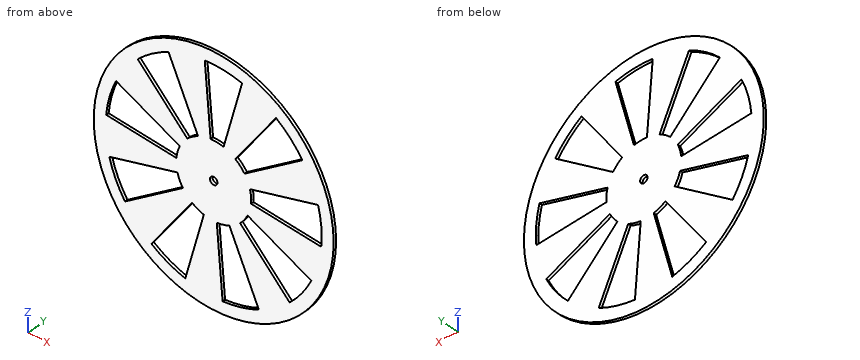
```python
from build123d import *

# Parameters (mm, degrees)
F0_R     = 50.8
F0_R_2   = 1.5875
F1_DEPTH = 1.1938


with BuildPart() as f1:
    # F0 (on Front) → F1 (new body)
    with BuildSketch(Plane.XZ):
        Circle(F0_R)
        with BuildLine():
            ThreePointArc((44.21609, 11.629953), (45.342464, 5.863394), (45.72, 0))
            ThreePointArc((45.72, 0), (45.671777, -2.09932), (45.527211, -4.194212))
            ThreePointArc((45.527211, -4.194212), (44.107234, -12.03621), (41.34708, -19.512494))
            ThreePointArc((41.34708, -19.512494), (37.330616, -26.3959), (32.17988, -32.47728))
            ThreePointArc((32.17988, -32.47728), (26.051375, -37.571855), (19.131311, -41.524828))
            ThreePointArc((19.131311, -41.524828), (11.629953, -44.21609), (3.775225, -45.563868))
            ThreePointArc((3.775225, -45.563868), (-4.194212, -45.527211), (-12.03621, -44.107234))
            ThreePointArc((-12.03621, -44.107234), (-19.512494, -41.34708), (-26.3959, -37.330616))
            ThreePointArc((-26.3959, -37.330616), (-32.47728, -32.17988), (-37.571855, -26.051375))
            ThreePointArc((-37.571855, -26.051375), (-41.524828, -19.131311), (-44.21609, -11.629953))
            ThreePointArc((-44.21609, -11.629953), (-45.563868, -3.775225), (-45.527211, 4.194212))
            ThreePointArc((-45.527211, 4.194212), (-44.107234, 12.03621), (-41.34708, 19.512494))
            ThreePointArc((-41.34708, 19.512494), (-37.330616, 26.3959), (-32.17988, 32.47728))
            ThreePointArc((-32.17988, 32.47728), (-26.051375, 37.571855), (-19.131311, 41.524828))
            ThreePointArc((-19.131311, 41.524828), (-11.629953, 44.21609), (-3.775225, 45.563868))
            ThreePointArc((-3.775225, 45.563868), (4.194212, 45.527211), (12.03621, 44.107234))
            ThreePointArc((12.03621, 44.107234), (19.512494, 41.34708), (26.3959, 37.330616))
            ThreePointArc((26.3959, 37.330616), (32.47728, 32.17988), (37.571855, 26.051375))
            ThreePointArc((37.571855, 26.051375), (41.524828, 19.131311), (44.21609, 11.629953))
        make_face(mode=Mode.SUBTRACT)
        with BuildLine():
            Line((-15.80806, 1.456324), (-45.527211, 4.194212))
            ThreePointArc((-45.527211, 4.194212), (-45.563868, -3.775225), (-44.21609, -11.629953))
            Line((-44.21609, -11.629953), (-15.352809, -4.038178))
            ThreePointArc((-15.352809, -4.038178), (-15.820788, -1.310842), (-15.80806, 1.456324))
        make_face()
        with BuildLine():
            Line((-11.173569, 11.276833), (-32.17988, 32.47728))
            ThreePointArc((-32.17988, 32.47728), (-37.330616, 26.3959), (-41.34708, 19.512494))
            Line((-41.34708, 19.512494), (-14.356625, 6.775171))
            ThreePointArc((-14.356625, 6.775171), (-12.962019, 9.165243), (-11.173569, 11.276833))
        make_face()
        with BuildLine():
            Line((-1.310842, 15.820788), (-3.775225, 45.563868))
            ThreePointArc((-3.775225, 45.563868), (-11.629953, 44.21609), (-19.131311, 41.524828))
            Line((-19.131311, 41.524828), (-6.642816, 14.418343))
            ThreePointArc((-6.642816, 14.418343), (-4.038178, 15.352809), (-1.310842, 15.820788))
        make_face()
        with BuildLine():
            Line((9.165243, 12.962019), (26.3959, 37.330616))
            ThreePointArc((26.3959, 37.330616), (19.512494, 41.34708), (12.03621, 44.107234))
            Line((12.03621, 44.107234), (4.17924, 15.315012))
            ThreePointArc((4.17924, 15.315012), (6.775171, 14.356625), (9.165243, 12.962019))
        make_face()
        with BuildLine():
            Line((15.352809, 4.038178), (44.21609, 11.629953))
            ThreePointArc((44.21609, 11.629953), (41.524828, 19.131311), (37.571855, 26.051375))
            Line((37.571855, 26.051375), (13.045783, 9.045616))
            ThreePointArc((13.045783, 9.045616), (14.418343, 6.642816), (15.352809, 4.038178))
        make_face()
        with BuildLine():
            ThreePointArc((41.34708, -19.512494), (44.107234, -12.03621), (45.527211, -4.194212))
            Line((45.527211, -4.194212), (15.80806, -1.456324))
            ThreePointArc((15.80806, -1.456324), (15.315012, -4.17924), (14.356625, -6.775171))
            Line((14.356625, -6.775171), (41.34708, -19.512494))
        make_face()
        with BuildLine():
            ThreePointArc((19.131311, -41.524828), (26.051375, -37.571855), (32.17988, -32.47728))
            Line((32.17988, -32.47728), (11.173569, -11.276833))
            ThreePointArc((11.173569, -11.276833), (9.045616, -13.045783), (6.642816, -14.418343))
            Line((6.642816, -14.418343), (19.131311, -41.524828))
        make_face()
        with BuildLine():
            ThreePointArc((-12.03621, -44.107234), (-4.194212, -45.527211), (3.775225, -45.563868))
            Line((3.775225, -45.563868), (1.310842, -15.820788))
            ThreePointArc((1.310842, -15.820788), (-1.456324, -15.80806), (-4.17924, -15.315012))
            Line((-4.17924, -15.315012), (-12.03621, -44.107234))
        make_face()
        with BuildLine():
            ThreePointArc((-37.571855, -26.051375), (-32.47728, -32.17988), (-26.3959, -37.330616))
            Line((-26.3959, -37.330616), (-9.165243, -12.962019))
            ThreePointArc((-9.165243, -12.962019), (-11.276833, -11.173569), (-13.045783, -9.045616))
            Line((-13.045783, -9.045616), (-37.571855, -26.051375))
        make_face()
        with BuildLine():
            ThreePointArc((15.875, 0), (15.743911, 2.035901), (15.352809, 4.038178))
            ThreePointArc((15.352809, 4.038178), (14.418343, 6.642816), (13.045783, 9.045616))
            ThreePointArc((13.045783, 9.045616), (11.276833, 11.173569), (9.165243, 12.962019))
            ThreePointArc((9.165243, 12.962019), (6.775171, 14.356625), (4.17924, 15.315012))
            ThreePointArc((4.17924, 15.315012), (1.456324, 15.80806), (-1.310842, 15.820788))
            ThreePointArc((-1.310842, 15.820788), (-4.038178, 15.352809), (-6.642816, 14.418343))
            ThreePointArc((-6.642816, 14.418343), (-9.045616, 13.045783), (-11.173569, 11.276833))
            ThreePointArc((-11.173569, 11.276833), (-12.962019, 9.165243), (-14.356625, 6.775171))
            ThreePointArc((-14.356625, 6.775171), (-15.315012, 4.17924), (-15.80806, 1.456324))
            ThreePointArc((-15.80806, 1.456324), (-15.820788, -1.310842), (-15.352809, -4.038178))
            ThreePointArc((-15.352809, -4.038178), (-14.418343, -6.642816), (-13.045783, -9.045616))
            ThreePointArc((-13.045783, -9.045616), (-11.276833, -11.173569), (-9.165243, -12.962019))
            ThreePointArc((-9.165243, -12.962019), (-6.775171, -14.356625), (-4.17924, -15.315012))
            ThreePointArc((-4.17924, -15.315012), (-1.456324, -15.80806), (1.310842, -15.820788))
            ThreePointArc((1.310842, -15.820788), (4.038178, -15.352809), (6.642816, -14.418343))
            ThreePointArc((6.642816, -14.418343), (9.045616, -13.045783), (11.173569, -11.276833))
            ThreePointArc((11.173569, -11.276833), (12.962019, -9.165243), (14.356625, -6.775171))
            ThreePointArc((14.356625, -6.775171), (15.315012, -4.17924), (15.80806, -1.456324))
            ThreePointArc((15.80806, -1.456324), (15.858256, -0.728931), (15.875, 0))
        make_face()
        Circle(F0_R_2, mode=Mode.SUBTRACT)
    extrude(amount=F1_DEPTH)


solid = f1.part
```
Part model, mm, in its own coordinate system. Round coordinates to 2 decimals unless told otherwise and drop trailing zeros. Order: outer loops, then holes, each group sorted by start corner. A loop starts at its lowest first (then second) coordinate and runs counter-clockwise, first axis right, second up. Notation, with made-up numbers: M 12,28 L 23,28 A8 ccw 23,41 Z; hole C -14,8 d8. An arc over 180 degrees is marked long. Answer in a Markdown table with one row per item. Add a question column.
Q1. Cut at D-D on z = 29.5. Give the cut face in (x, y).
Q2. Cut at B-B on z = -28. Give the cut face in (x, y).
Q3. Cut at C-C on y = -0.7. Give the number of separate pieces and of enclosed holes in the cut face, and give its area (3 significant figures).
Q4. Cut at A-A on x = 0. Give the cut face in (y, z) (1 decimal).
Q5. Wall check: L1, parallel to Z at x = 0, y = -0.3 (1 decimal); L2, parallel to X at y = -0.05, z = 12; L3, parallel to Z at x = -36, y = -1.1. Give the ranges that are in metal, low to high. Write a range as from..to.
Established:
| question | item | result |
|---|---|---|
| 1 | outline | M -41.36,-1.19 L -29.23,-1.19 L -29.23,0 L -41.36,0 Z; M -13.59,-1.19 L -2.44,-1.19 L -2.44,0 L -13.59,0 Z; M 8.05,-1.19 L 20.86,-1.19 L 20.86,0 L 8.05,0 Z; M 34.93,-1.19 L 41.36,-1.19 L 41.36,0 L 34.93,0 Z |
| 2 | outline | M -42.39,-1.19 L -19.8,-1.19 L -19.8,0 L -42.39,0 Z; M -7.64,-1.19 L 2.32,-1.19 L 2.32,0 L -7.64,0 Z; M 12.9,-1.19 L 27.74,-1.19 L 27.74,0 L 12.9,0 Z; M 36.14,-1.19 L 42.39,-1.19 L 42.39,0 L 36.14,0 Z |
| 3 | separate pieces | 1 |
| 3 | enclosed holes | 10 |
| 3 | area | 5,210 mm2 |
| 4 | outline | M -1.2,-50.8 L 0,-50.8 L 0,-1.6 L -1.2,-1.6 Z; M -1.2,1.6 L 0,1.6 L 0,15.9 L -1.2,15.9 Z; M -1.2,45.7 L 0,45.7 L 0,50.8 L -1.2,50.8 Z |
| 5 | L1 | z = -50.8..-1.6, 1.6..15.9, 45.7..50.8 |
| 5 | L2 | x = -49.36..-44.12, -25.43..-11.89, -10.39..10.39, 17.31..49.36 |
| 5 | L3 | z = -35.84..-24.96, -9.47..3.32, 16.99..35.84 |
